Could you check a few things on this model? Use its own coordinates, in mm. A direction names the side the tool comes from. Give positions to 0.01 mm unless a question says otherwise; leave off trailing zeros. Order: outer loops, then holes, each group sorted by start corner. A loop starts at its lowest first (then second) coordinate and runs counter-clockwise, first axis right, second up. Notation, with made-up numbers: (80, 59.5) - (96, 59.5) arc R12 ccw to (96, 74.5) - close; hole circle Ø3 at (-16, 30). An arc over 180 degrees is marked (long way). Put each result on its own line as item: value.
from build123d import *

# Parameters (mm, degrees)
BOSS_EXTRUDE1_DEPTH = 10
SKETCH4_R           = 1.5
SKETCH4_R_2         = 0.8
CUT_EXTRUDE1_DEPTH  = 42
SKETCH6_R           = 0.8
CUT_EXTRUDE2_DEPTH  = 26
CUT_EXTRUDE3_DEPTH  = 2
SKETCH9_R           = 2.5
CUT_EXTRUDE4_DEPTH  = 10


with BuildPart() as part:
    # Sketch2 → Boss-Extrude1 (new body)
    with BuildSketch(Plane.XY):
        Polygon((-16.5, -11), (-19.5, -11), (-19.5, 14), (21.5, 14), (21.5, -11), (16.5, -11), (16.5, 11), (-16.5, 11), align=None)
    extrude(amount=BOSS_EXTRUDE1_DEPTH)

    # Sketch4 → Cut-Extrude1 (cut, through all)
    with BuildSketch(Plane.ZY.offset(19.5)):
        with Locations((5, -6)):
            Circle(SKETCH4_R)
        with Locations((5, -1)):
            Circle(SKETCH4_R_2)
    extrude(amount=-CUT_EXTRUDE1_DEPTH, mode=Mode.SUBTRACT)

    # Sketch6 → Cut-Extrude2 (cut, through all)
    with BuildSketch(Plane(origin=(0, 14, 0), x_dir=(1, 0, 0), z_dir=(0, 1, 0))):
        with Locations((-7, -5)):
            Circle(SKETCH6_R)
        with Locations((11, -5)):
            Circle(SKETCH6_R)
        with Locations((5, -5)):
            Circle(SKETCH6_R)
    extrude(amount=-CUT_EXTRUDE2_DEPTH, mode=Mode.SUBTRACT)

    # Sketch8 → Cut-Extrude3 (cut)
    with BuildSketch(Plane.ZY.offset(-16.5)):
        Polygon((1, -1), (1, -11), (9, -11), (9, -1), (7, 12), (3, 12), align=None)
    extrude(amount=-CUT_EXTRUDE3_DEPTH, mode=Mode.SUBTRACT)

    # Sketch9 → Cut-Extrude4 (cut)
    with BuildSketch(Plane.ZY.offset(19.5)):
        with Locations((5, -6)):
            Circle(SKETCH9_R)
    extrude(amount=-CUT_EXTRUDE4_DEPTH, mode=Mode.SUBTRACT)


solid = part.part
1) Which directions (+Z, -Z, +X, -X, +Y, -Y) give clear straight access to the entire face, cutting with the end or side of a thin tool? Please do faces 4 (the flat face through (4, 12, 0)), 5 (the flat face through (17.486, 5.409, 8.014)), 6 (the flat face through (16.5, 2, 9)).
Filled in:
face 4: -Z, +X, -X, +Y, -Y
face 5: -Y
face 6: +Z, -Z, -Y
2) We'd pull the mould along Y, two halves only. Please class faces 1 (the flat face through (-19.5, 1, 5)), 2 (the flat face through (0, 11, 5)), 3 (the cylindrical face through (19.979, -6.575, 6.386)): pulls with the +Y half, pulls with the -Y half, needs draft (parallel to the pull), parting line crosses it, or undercut.
Filled in:
face 1: needs draft
face 2: pulls with the -Y half
face 3: undercut
3) Suppose I cut it at B-B, the plane x = 11. List the corners of the cut face in (y, z) for me.
Filled in:
outline: (11, 0) - (14, 0) - (14, 4.2) - (11, 4.2) - close; (11, 5.8) - (14, 5.8) - (14, 10) - (11, 10) - close
4) I'm going to push flat-ended pins straight in: pin 1 (1.8 mm diameter, centred on y = -1, z = 5, fed in from -X); pin 2 (2 mm diameter, centred on x = 5, z = 5, fed in from -Y). Where does each tip first touch, or does it pass through?
Filled in:
pin 1: stops at x = -19.5
pin 2: stops at y = 11
5) Suppose I cut it at C-C, the plane y = -9.25. List the corners of the cut face in (x, z) for me.
Filled in:
outline: (-19.5, 0) - (-16.5, 0) - (-16.5, 10) - (-19.5, 10) - close; (16.5, 0) - (21.5, 0) - (21.5, 10) - (16.5, 10) - (16.5, 9) - (18.5, 9) - (18.5, 1) - (16.5, 1) - close
6) If I drill on line 1 (Y direction, x = 20.65, z = 5); line 2 (Y direction, x = -17.8, z = 5); line 3 (X direction, y = 2, z = 5.5), over which ranges is the centre line in solid material (lowest first)? Write a range as [from, to].
Filled in:
line 1: y = [-11, -7.5], [-4.5, -1.8], [-0.2, 14]
line 2: y = [-11, -8.5], [-3.5, -1.8], [-0.2, 14]
line 3: x = [-19.5, -16.5], [18.5, 21.5]
7) Suppose I cut it at A-A, the plane y = -6. List the corners of the cut face in (x, z) for me.
Filled in:
outline: (-19.5, 0) - (-16.5, 0) - (-16.5, 2.5) - (-19.5, 2.5) - close; (-19.5, 7.5) - (-16.5, 7.5) - (-16.5, 10) - (-19.5, 10) - close; (16.5, 0) - (21.5, 0) - (21.5, 3.5) - (18.5, 3.5) - (18.5, 1) - (16.5, 1) - close; (16.5, 9) - (18.5, 9) - (18.5, 6.5) - (21.5, 6.5) - (21.5, 10) - (16.5, 10) - close
8) Suppose I cut it at D-D, the plane z = 5. State how many separate pieces and enclosed holes the cut face has, and give its area (3 significant figures).
Filled in:
separate pieces: 8
enclosed holes: 0
area: 205 mm^2
